from build123d import *

# Parameters (mm, degrees)
F1_DEPTH = 6.35
F2_SIZE2 = 3.81
F2_SIZE  = 7.112


with BuildPart() as f1:
    # F0 (on Right) → F1 (new body)
    with BuildSketch(Plane.YZ):
        Polygon((26.7912242562, 26.1120563269), (1.3912242562, 26.1120563269), (1.3912242562, -50.0879436731), (26.7912242562, -50.0879436731), (26.7912242562, 3.7854563269), (26.7912242562, 9.8814563269), align=None)
        with BuildLine():
            ThreePointArc((10.1224742562, 15.7933063269), (14.0912242562, 19.7620563269), (18.0599742562, 15.7933063269))
            Line((18.0599742562, 15.7933063269), (18.0599742562, -1.6691936731))
            ThreePointArc((18.0599742562, -1.6691936731), (14.0912242562, -5.6379436731), (10.1224742562, -1.6691936731))
            Line((10.1224742562, -1.6691936731), (10.1224742562, 15.7933063269))
        make_face(mode=Mode.SUBTRACT)
    extrude(amount=F1_DEPTH)

    # F2
    f2_edges = [f1.edges().sort_by_distance(p)[0] for p in [
        (3.175, 1.391224, -50.087944),
        (3.175, 26.791224, -50.087944),
    ]]
    f2_side = f1.faces().sort_by_distance((3.175, 14.091224, -50.087944))[0]
    chamfer(f2_edges, length=F2_SIZE, length2=F2_SIZE2, reference=f2_side)


solid = f1.part
Can you work these out from the model? Positions are in its coordinate system, mm. A direction names the side the tool comes from. Round coordinates to 2 decimals unless told otherwise and drop trailing zeros. Order: outer loops, then holes, each group sorted by start corner. A loop starts at its lowest first (then second) coordinate and runs counter-clockwise, first axis right, second up. Notation, with made-up numbers: (7, -1) -> (29, -1) arc R28 ccw to (29, 25) -> close; hole circle Ø8 at (19.25, -29.75). An arc over 180 degrees is marked (long way). Write each question's results on one line, items separated by ' | '. Start each with the question number.
Item 1: If we section it at C-C, the plane x = 1.25: Write out the boundary of the cut face in (y, z).
Item 2: Please list where these lines run through material, in increasing order: L1, parallel to Y at x = 3.5, z = 12; L2, parallel to Z at x = 3, y = 16.25; L3, parallel to Z at x = 6.25, y = 15.
Item 3: If we section it at B-B, the plane y = 17.25: Write out the boundary of the cut face in (x, z).
Item 4: Thinking about a two-plate mould opening in Y: for faces 3 (the flat face through (3, 14, -50.088)), 4 (the flat face through (3.131, 4.897, -48.156)), 5 (the flat face through (3, 10.122, 7)), which applies, +Y half, -Y half, draft (parallel to the pull), parting line (faces both ways), or undercut?
Item 5: Which directions (+Z, -Z, +X, -X, +Y, -Y) give clear straight access to the entire face, cutting with the end or side of a thin tool? Please do faces 1 (the flat face through (0, 14, -11)), 2 (the cylindrical face through (3.13, 14, 19.76)).
Item 6: If we section it at A-A, the plane z = 4.5: Write out the boundary of the cut face in (x, y).
Item 7: If we section it at D-D, the plane y = 4.75: Write out the boundary of the cut face in (x, z), then the cut area to 3 significant figures.
Results:
1) outline: (1.39, -46.28) -> (8.5, -50.09) -> (19.68, -50.09) -> (26.79, -46.28) -> (26.79, 26.11) -> (1.39, 26.11) -> close; hole (10.12, -1.67) arc R3.97 ccw to (18.06, -1.67) -> (18.06, 15.79) arc R3.97 ccw to (10.12, 15.79) -> close
2) L1: y = 1.39 to 10.12, 18.06 to 26.79 | L2: z = -50.09 to -5, 19.12 to 26.11 | L3: z = -50.09 to -5.53, 19.66 to 26.11
3) outline: (0, -50.09) -> (6.35, -50.09) -> (6.35, -4.07) -> (0, -4.07) -> close; (0, 18.2) -> (6.35, 18.2) -> (6.35, 26.11) -> (0, 26.11) -> close
4) face 3: draft | face 4: -Y half | face 5: undercut
5) face 1: +Z, -Z, -X, +Y, -Y | face 2: +X, -X
6) outline: (0, 1.39) -> (6.35, 1.39) -> (6.35, 10.12) -> (0, 10.12) -> close; (0, 18.06) -> (6.35, 18.06) -> (6.35, 26.79) -> (0, 26.79) -> close
7) outline: (0, -48.08) -> (6.35, -48.08) -> (6.35, 26.11) -> (0, 26.11) -> close | area: 471 mm2
